Read the model definition and answer for the solid it produces. Units are mm, in the model's axes. Face numbers are marked on the shaded views. A direction names the side the tool comes from. Coordinates: 2 decimals unless noted, no trailing zeros. Loops run counter-clockwise (first coordinate to the right, second up) from the corner with the lowest first, then second, coordinate; pieces in that order, holes last.
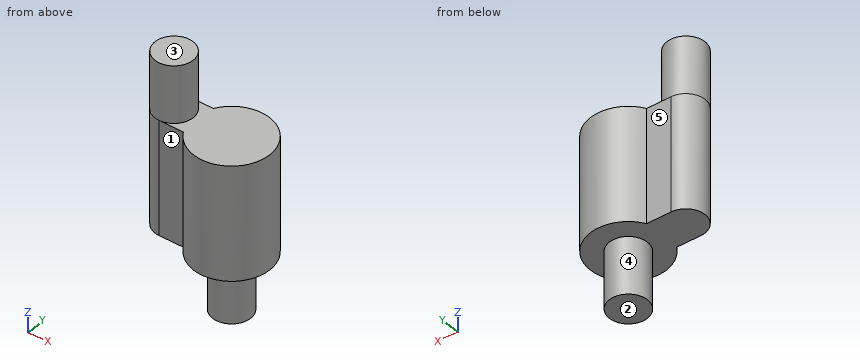
from build123d import *

# Parameters (mm, degrees)
BOSS_EXTRUDE1_DEPTH = 6
SKETCH2_R           = 1
BOSS_EXTRUDE2_DEPTH = 3
SKETCH3_R           = 1
BOSS_EXTRUDE3_DEPTH = 3


with BuildPart() as part:
    # Sketch1 → Boss-Extrude1 (new body)
    with BuildSketch(Plane.XY):
        with BuildLine():
            Line((-7.068000803, 8.031631057), (-5.800051611, 8.031631057))
            ThreePointArc((-5.800051611, 8.031631057), (-2.068000803, 7.031631057), (-5.800051611, 6.031631057))
            Line((-5.800051611, 6.031631057), (-7.068000803, 6.031631057))
            ThreePointArc((-7.068000803, 6.031631057), (-8.068000803, 7.031631057), (-7.068000803, 8.031631057))
        make_face()
    extrude(amount=BOSS_EXTRUDE1_DEPTH)

    # Sketch2 → Boss-Extrude2 (add)
    with BuildSketch(Plane.XY.offset(6)):
        with Locations((-7.068000803, 7.031631057)):
            Circle(SKETCH2_R)
    extrude(amount=BOSS_EXTRUDE2_DEPTH)

    # Sketch3 → Boss-Extrude3 (add)
    with BuildSketch(Plane(origin=(0, 0, 0), x_dir=(-1, 0, 0), z_dir=(0, 0, -1))):
        with Locations((4.068000803, 7.031631057)):
            Circle(SKETCH3_R)
    extrude(amount=BOSS_EXTRUDE3_DEPTH)


solid = part.part
Q1. Which of the six approach directions +Z, -Z, +X, -X, +Y, -Y give full straight-line access (tool end or side, diameter ignored) to the marked faces 1, 2, 3, 4 and 5?
Findings below:
face 1: +Z, -Z, -X, -Y
face 2: -Z, +X, -X, +Y, -Y
face 3: +Z, +X, -X, +Y, -Y
face 4: -Z
face 5: +Z, -Z, -X, +Y
Q2. A cutting plane is placed at C-C (z = 3.5). Give the vertices of the cut face in (x, y), then the cut area to 3 significant figures.
Findings below:
outline: (-7.07, 6.03) - (-5.8, 6.03) arc R2 ccw (long way) to (-5.8, 8.03) - (-7.07, 8.03) arc R1 ccw to start
area: 16.3 mm2
Q3. A cutting plane is placed at D-D (x = -3.9). Give the vertices of the cut face in (y, z).
Findings below:
outline: (5.04, 0) - (6.05, 0) - (6.05, -3) - (8.02, -3) - (8.02, 0) - (9.02, 0) - (9.02, 6) - (5.04, 6) - close
Q4. Straight lines are drawn through the part: probe 1 along Z at (x, y) = (-4.9, 6.8); probe 2 along X at (y, z) = (7.1, -0.75); probe 3 along X at (y, z) = (7.1, 0.25). For each, find the intervals that lie inside material, in ascending order.
Findings below:
probe 1: z = -3 to 6
probe 2: x = -5.07 to -3.07
probe 3: x = -8.07 to -2.07
Q5. A cutting plane is placed at B-B (x = -5.95). Give the vertices of the cut face in (y, z), then the cut area to 3 significant figures.
Findings below:
outline: (6.03, 0) - (8.03, 0) - (8.03, 6) - (6.03, 6) - close
area: 12.0 mm2
Q6. A cutting plane is placed at A-A (y = 6.75). Give the vertices of the cut face in (x, z), then the cut area to 3 significant figures.
Findings below:
outline: (-8.03, 0) - (-5.03, 0) - (-5.03, -3) - (-3.11, -3) - (-3.11, 0) - (-2.09, 0) - (-2.09, 6) - (-6.11, 6) - (-6.11, 9) - (-8.03, 9) - close
area: 47.2 mm2
